```python
from build123d import *

# Parameters (mm, degrees)
SKETCH1_R           = 4
BOSS_EXTRUDE1_DEPTH = 65.5
SKETCH2_R           = 1
CUT_EXTRUDE1_DEPTH  = 66.5
SKETCH3_R           = 3.14325
CUT_EXTRUDE2_DEPTH  = 9.0297
CUT_EXTRUDE2_TAPER  = 2.328
SKETCH4_R           = 3.14325
CUT_EXTRUDE3_DEPTH  = 9.0297
CUT_EXTRUDE3_TAPER  = 2.328


with BuildPart() as part:
    # Sketch1 → Boss-Extrude1 (new body)
    with BuildSketch(Plane.XY):
        Circle(SKETCH1_R)
    extrude(amount=BOSS_EXTRUDE1_DEPTH)

    # Sketch2 → Cut-Extrude1 (cut, through all)
    with BuildSketch(Plane.XY):
        Circle(SKETCH2_R)
    extrude(amount=CUT_EXTRUDE1_DEPTH, mode=Mode.SUBTRACT)

    # Sketch3 → Cut-Extrude2 (cut)
    with BuildSketch(Plane.XY):
        Circle(SKETCH3_R)
    extrude(amount=CUT_EXTRUDE2_DEPTH, taper=CUT_EXTRUDE2_TAPER, mode=Mode.SUBTRACT)

    # Sketch4 → Cut-Extrude3 (cut)
    with BuildSketch(Plane.XY.offset(65.5)):
        Circle(SKETCH4_R)
    extrude(amount=-CUT_EXTRUDE3_DEPTH, taper=CUT_EXTRUDE3_TAPER, mode=Mode.SUBTRACT)


solid = part.part
```
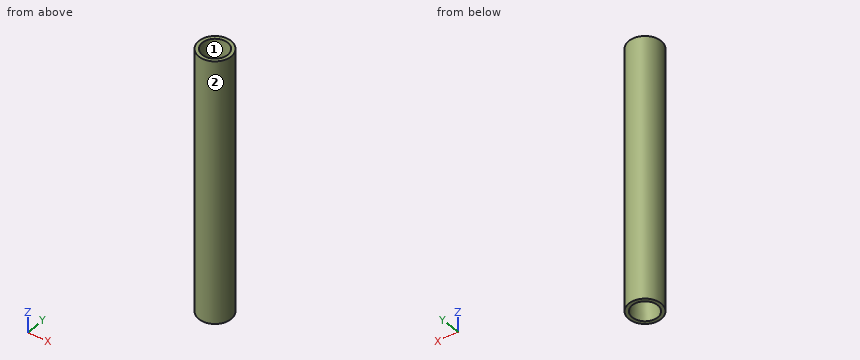
Build history of the part. All positions in model axes, mm. Face numbers are marked on the shaded views. Round coordinates to 2 decimals unless told otherwise and drop trailing zeros. Order: outer loops, then holes, each group sorted by start corner. A loop starts at its lowest first (then second) coordinate and runs counter-clockwise, first axis right, second up. Notation, with made-up numbers: (-31, -6.75) - (0, -6.75) arc R22 ccw to (0, 22.25) - close; hole circle Ø6 at (17.5, 53). An arc over 180 degrees is marked (long way). Use a Markdown table: item, result.
1) Pull direction Y, two halves, no side cores. Call the marked faces 1 and 2: pulls with the +Y half, pulls with the -Y half, needs draft (parallel to the pull), parting line crosses it, or undercut.
Recorded:
| item | result |
|---|---|
| face 1 | undercut |
| face 2 | parting line crosses it |
2) Wall check: L1, parallel to Y at x = 0, z = 21; L2, parallel to Z at x = 1.5, y = -2.25; L3, parallel to X at y = 0.5, z = 17. Give the ranges that are in metal, low to high.
Recorded:
| item | result |
|---|---|
| L1 | y = -4 to -1, 1 to 4 |
| L2 | z = 9.03 to 56.47 |
| L3 | x = -3.97 to -0.87, 0.87 to 3.97 |
3) Saw through at B-B on z = 30. Write the cut outline in (x, y), and give its area (3 significant figures).
Recorded:
| item | result |
|---|---|
| outline | circle Ø8 at (0, 0); hole circle Ø2 at (0, 0) |
| area | 47.1 mm² |
4) Flat gauge pins, fed straight in: pin 1 Ø3 at (x, y) = (0, 0) entering from +Z; pin 2 Ø4 at (y, z) = (-1.5, 22.5) entering from -X; pin 3 Ø2 at (y, z) = (3, 18) entering from -X. Where does each tip first touch, or does it go through?
Recorded:
| item | result |
|---|---|
| pin 1 | stops at z = 56.47 |
| pin 2 | stops at x = -4 |
| pin 3 | stops at x = -3.46 |
5) Saw through at A-A on x = 0. Write the cut outline in (y, z), and give its area (3 significant figures).
Recorded:
| item | result |
|---|---|
| outline | (-4, 0) - (-3.14, 0) - (-2.78, 9.03) - (-1, 9.03) - (-1, 56.47) - (-2.78, 56.47) - (-3.14, 65.5) - (-4, 65.5) - close; (1, 9.03) - (2.78, 9.03) - (3.14, 0) - (4, 0) - (4, 65.5) - (3.14, 65.5) - (2.78, 56.47) - (1, 56.47) - close |
| area | 322 mm² |
